from build123d import *

# Parameters (mm, degrees)
F1_DEPTH = 15
F2_T     = -1.2
F3_R     = 1.2


with BuildPart() as f1:
    # F0 (on Right) → F1 (new body, symmetric)
    with BuildSketch(Plane.YZ):
        Polygon((-2.9243966283, 0.669256573), (0, 0), (0, 27), (-13, 27), (-27.3767851269, 0.669256573), (-15.3014834083, -14), (-1.1154276217, -18.8739943805), (0, -14), (-2.9243966283, -13.330743427), align=None)
    extrude(amount=F1_DEPTH, both=True)

    # F2
    f2_openings = [f1.faces().sort_by_distance(p)[0] for p in [
        (0, 0, 13.5),
        (0, -0.557714, -16.436997),
        (0, -20.188393, 13.834628),
    ]]
    offset(amount=F2_T, openings=f2_openings, kind=Kind.INTERSECTION)

    # F3
    f3_edges = [f1.edges().sort_by_distance(p)[0] for p in [
        (-15, -6.5, 27),
        (15, -6.5, 27),
        (-15, -8.208456, -16.436997),
        (0, -15.301483, -14),
        (-15, -21.339134, -6.665372),
        (15, -8.208456, -16.436997),
        (15, -21.339134, -6.665372),
    ]]
    fillet(f3_edges, radius=F3_R)


solid = f1.part
Can you work these out from the model? Positions are in its coordinate system, mm. A direction names the side the tool comes from. Give positions to 0.01 mm unless a question says otherwise; leave off trailing zeros. Write each loop counter-clockwise with the first axis right and the second up, starting at its lowest first coordinate (ties: lowest second). Pieces come first, ordered by that corner, then holes. Notation, with made-up numbers: M 15,23.25 L 29,23.25 A10 ccw 29,31.25 Z; hole C -12,18.5 d5. An arc over 180 degrees is marked long. Answer in a Markdown table with one row per item. Add a question column.
Item 1: We'd pull the mould along Z, two halves only. Please class faces 6 (the flat face through (0.21, -1.44, -13.67)), 7 (the flat face through (0.193, -8.145, -16.459)), 8 (the flat face through (0.19, -20.76, -5.48)): released by +Z, released by -Z, zero draft, split by the parting line, or undercut.
Item 2: For pin 1 Ø12 at (x, y) = (10.5, -12) entering from -Z; pin 2 Ø1 at (y, z) = (-16, -12) entering from -X; pin 3 Ø1 at (x, y) = (-2.5, -16) entering from -Z; pin 4 Ø7 at (x, y) = (2, -7) entering from -Z, each with a flat end and sliding along its axis, tell me the tip position at first contact or that it passes through.
Item 3: Imagine slicing it at D-D, the plane z = 14.5. Write out the boundary of the cut face in (x, y), plus the area to 3 significant figures.
Item 4: Please list where these lines run through material, in increasing order: L1, parallel to X at y = -13, z = 23.5; L2, parallel to Z at x = -12, y = -2.5; L3, parallel to Z at x = -12.5, y = -3.5.
Item 5: Imagine slicing it at C-C, the plane y = -1.75. State how many separate pieces and enclosed holes the cut face has, plus the area to 3 significant figures.
Item 6: Imagine slicing it at A-A, the plane x = 5. Write out the boundary of the cut face in (y, z), plus the area to 3 significant figures.
Item 7: On a 3-axis mill with a long thin cutter (end or side, diameter ignored), from which of +Z, -Z, +X, -X, +Y, -Y can I reach the whole of each face in a straight line? I mean faces 1 (the flat face through (-13.8, -11, 4)), 2 (the flat face through (0, -7, 25.8)), 3 (the flat face through (0.19, -2.09, 1.71)), 4 (the flat face through (-15, -11, 4)), 5 (the cylindrical face through (14.658, -7.834, -16.184)). Say none if no direction works.
Item 8: Imagine slicing it at B-B, the plane z = 24. Write out the boundary of the cut face in (x, y).
Evaluation:
| question | item | result |
|---|---|---|
| 1 | face 6 | undercut |
| 1 | face 7 | released by -Z |
| 1 | face 8 | released by +Z |
| 2 | pin 1 | stops at z = -17.2 |
| 2 | pin 2 | stops at x = -15 |
| 2 | pin 3 | stops at z = -13.76 |
| 2 | pin 4 | stops at z = -18.05 |
| 3 | outline | M -15,-19.83 L -13.8,-19.83 L -13.8,0 L -15,0 Z; M 13.8,-19.83 L 15,-19.83 L 15,0 L 13.8,0 Z |
| 3 | area | 47.6 mm² |
| 4 | L1 | x = -15 to -13.8, 13.8 to 15 |
| 4 | L2 | z = -18.4 to -17.13, -14.66 to -13.43, 0.57 to 1.8, 25.8 to 27 |
| 4 | L3 | z = -18.05 to -16.79, -14.43 to 2.03, 25.8 to 27 |
| 5 | separate pieces | 2 |
| 5 | enclosed holes | 2 |
| 5 | area | 211 mm² |
| 6 | outline | M -27.38,0.67 L -15.52,-13.74 A1.2 ccw -14.98,-14.11 L -1.12,-18.87 L -0.85,-17.7 L -14.59,-12.98 L -26.76,1.8 Z; M -13.66,25.8 L 0,25.8 L 0,27 L -13,27 Z; M -4.12,-14.29 L -0.27,-15.17 L 0,-14 L -2.92,-13.33 L -2.92,0.67 L 0,0 L 0,1.23 L -4.12,2.17 Z |
| 6 | area | 83.4 mm² |
| 7 | face 1 | none |
| 7 | face 2 | +Y, -Y |
| 7 | face 3 | +Y |
| 7 | face 4 | +Z, -Z, -X, +Y, -Y |
| 7 | face 5 | -Z, +X, -Y |
| 8 | outline | M -15,-14.64 L -13.8,-14.64 L -13.8,0 L -15,0 Z; M 13.8,-14.64 L 15,-14.64 L 15,0 L 13.8,0 Z |
